Autodesk Inventor part; units mm, degrees
ref_plane "Work Plane2" through (0, 17.6708, -22.228) normal (0, 0, -1) x (0, 1, 0)
ref_plane "YZ Plane" through (0, 0, 0) normal (1, 0, 0) x (0, 1, 0)
ref_plane "XZ Plane" through (0, 0, 0) normal (0, 1, 0) x (-1, 0, 0)
ref_plane "Work Plane1" through (0, 0, 0) normal (0, 0, 1) x (1, 0, 0)
sketch "Sketch1" plane through (0, 0, 0) normal (0, 0, 1) x (1, 0, 0)
  arc A0 (18.9992, 41.108) -> (0, 60.0877) centre (-0.0008, 41.0877) ccw construction
  arc A1 (0, 22.1284) -> (18.9992, 41.108) centre (-0.0008, 41.1284) ccw construction
  arc A2 (44.3468, 60.0877) -> (25.3476, 41.108) centre (44.3476, 41.0877) ccw construction
  arc A3 (25.3476, 41.108) -> (44.3468, 22.1284) centre (44.3476, 41.1284) ccw construction
  line L0 (10.16, 73.6386) -> (5.7912, 73.6386) construction
  line L1 (0, 77.677) -> (0, 67.7202) construction
  line L2 (5.7912, 73.6386) -> (13.9012, 73.6386) construction
  line L3 (-25.35, 77.677) -> (-25.35, 84.027)
  line L4 (-25.35, -6.35) -> (-25.35, 0)
  line L5 (-25.35, 77.677) -> (-25.35, 0) construction
  arc A4 (-6.0324, 64.4924) -> (-6.0325, 17.7644) centre (-0.0008, 41.1284) ccw
  arc A5 (-6.0324, 64.4924) -> (-6.0325, 17.7644) centre (-0.0008, 41.1284) ccw
  arc A6 (-0.0008, 60.1276) -> (-0.0008, 22.1292) centre (-0.0008, 41.1284) ccw
  line L6 (-6.0324, 64.4924) -> (-6.0324, 73.6793)
  line L7 (10.16, 8.5775) -> (5.7912, 8.5775) construction
  line L8 (-6.0325, 8.5775) -> (-6.0325, 17.7644)
  line L9 (-0.0008, 73.6793) -> (-0.0008, 60.1276)
  line L10 (-0.0008, 8.5775) -> (-0.0008, 22.1292)
  line L11 (-6.0324, 73.6793) -> (-6.0324, 76.2193)
  line L12 (-6.0324, 76.2193) -> (0, 76.2193)
  line L13 (-0.0008, 73.6793) -> (0, 76.2193)
  line L14 (-6.0325, 8.5775) -> (-6.0325, 6.0375)
  line L15 (-6.0325, 6.0375) -> (-0.0008, 6.0375)
  line L16 (-0.0008, 6.0375) -> (-0.0008, 8.5775)
  point P0 (0, 0)
  dimension "d12" = 18.9992
  dimension "d13" = 24.13
  dimension "d19" = 6.0317
  dimension "d22" = 6.0317
  dimension "d23" = 0
  dimension "d24" = 0
  dimension "d44" = 2.54
  dimension "d45" = 2.54
ref_plane "Work Plane2" through (0, 17.6708, -22.228) normal (0, 0, -1) x (0, 1, 0)
extrude "Extrusion1" add sketch "Sketch1" against normal up to surface (22.228 mm away)
fillet "Fillet1" radius 3.175 1 edges at (-6.0324, 64.4924, -11.114)
fillet "Fillet2" radius 3.175 1 edges at (-6.0325, 17.7644, -11.114)
sketch "Sketch3" plane through (-6.0325, 8.5775, -22.228) normal (-1, 0, 0) x (0, 0, 1)
  circle A0 centre (5.08, 4.7016) radius 1.9304 construction
  circle A1 centre (17.148, 4.7016) radius 1.9304 construction
  circle A2 centre (17.148, 60.4409) radius 1.9304 construction
  circle A3 centre (5.08, 60.4409) radius 1.9304 construction
  line L0 (5.08, 4.0666) -> (5.08, 5.3366) construction
  line L1 (7.0104, 4.0666) -> (7.0104, 5.3366)
  line L2 (3.1496, 5.3366) -> (3.1496, 4.0666)
  arc A4 (3.1496, 4.0666) -> (7.0104, 4.0666) centre (5.08, 4.0666) ccw
  arc A5 (7.0104, 5.3366) -> (3.1496, 5.3366) centre (5.08, 5.3366) ccw
  point P0 (22.228, -8.5775)
  point P1 (5.08, 7.9375)
  dimension "d25" = 0.635
  dimension "d26" = 0.635
  dimension "d27" = 3.8608
extrude "Extrusion3" cut sketch "Sketch3" against normal through all both and the other way through all
sketch "Sketch4" plane through (-6.0325, 8.5775, -22.228) normal (-1, 0, 0) x (0, 0, 1)
  circle A0 centre (17.148, 4.7016) radius 1.9304 construction
  circle A1 centre (5.08, 60.4409) radius 1.9304 construction
  circle A2 centre (17.148, 60.4409) radius 1.9304 construction
  line L0 (17.148, 4.0666) -> (17.148, 5.3366) construction
  line L1 (19.0784, 4.0666) -> (19.0784, 5.3366)
  line L2 (15.2176, 5.3366) -> (15.2176, 4.0666)
  arc A3 (15.2176, 4.0666) -> (19.0784, 4.0666) centre (17.148, 4.0666) ccw
  arc A4 (19.0784, 5.3366) -> (15.2176, 5.3366) centre (17.148, 5.3366) ccw
  line L3 (5.08, 59.8059) -> (5.08, 61.0759) construction
  line L4 (7.0104, 59.8059) -> (7.0104, 61.0759)
  line L5 (3.1496, 61.0759) -> (3.1496, 59.8059)
  arc A5 (3.1496, 59.8059) -> (7.0104, 59.8059) centre (5.08, 59.8059) ccw
  arc A6 (7.0104, 61.0759) -> (3.1496, 61.0759) centre (5.08, 61.0759) ccw
  line L6 (17.148, 59.8059) -> (17.148, 61.0759) construction
  line L7 (19.0784, 59.8059) -> (19.0784, 61.0759)
  line L8 (15.2176, 61.0759) -> (15.2176, 59.8059)
  arc A7 (15.2176, 59.8059) -> (19.0784, 59.8059) centre (17.148, 59.8059) ccw
  arc A8 (19.0784, 61.0759) -> (15.2176, 61.0759) centre (17.148, 61.0759) ccw
  point P0 (22.228, -8.5775)
  point P1 (17.148, 4.7016)
  dimension "d30" = 0.635
  dimension "d31" = 0.635
  dimension "d32" = 0.635
  dimension "d33" = 0.635
  dimension "d34" = 0.635
  dimension "d35" = 0.635
  dimension "d36" = 3.8608
  dimension "d37" = 3.8608
  dimension "d38" = 3.8608
extrude "Extrusion4" cut sketch "Sketch4" against normal through all both and the other way through all
equation "\"d19\" = d18"
properties part number "motor mount cap"
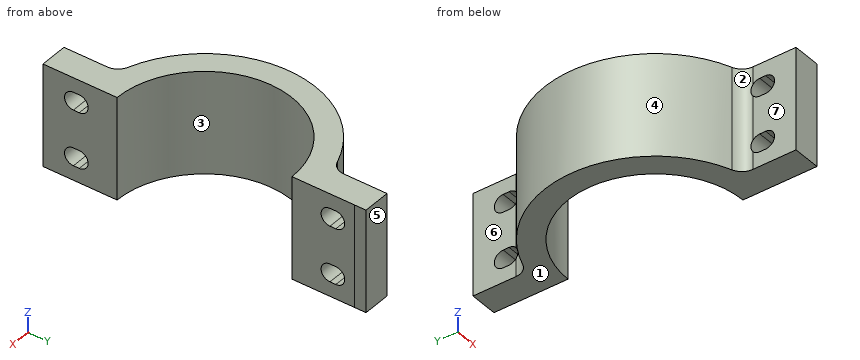
Read the model definition and answer for the solid it produces. Units are mm, in the model's axes. Face numbers are marked on the shaded views. A direction names the side the tool comes from. Round coordinates to 2 decimals unless told otherwise and drop trailing zeros. Order: outer loops, then holes, each group sorted by start corner. A loop starts at its lowest first (then second) coordinate and runs counter-clockwise, first axis right, second up. Notation, with made-up numbers: (60, -27.5) - (76, -27.5) arc R21 cw to (76, -9.5) - close; hole circle Ø10 at (-16.5, 17). An arc over 180 degrees is marked (long way). Use one line per item in the form item = value. Start each with the question number.
(1) Determine the mould class of the marked faces 1, 2, 3 and 4 for opening direction Y: +Y half, -Y half, draft (parallel to the pull), parting line (faces both ways), or undercut.
(2) For the marked faces 5, 6 and 7, determine the directions among +Z, -Z, +X, -X, +Y, -Y from which every point of the face is accessible in a straight line to the end or side of a thin tool.
(3) Flat-ended cylindrical pins translate along their axes: pin 1 Ø5 at (y, z) = (36, -2.5) entering from -X; pin 2 Ø7.5 at (y, z) = (72.5, -15) entering from -X; pin 3 Ø10 at (y, z) = (64, -20) entering from -X. Find the tip coordinate at first contact, or state that the pin passes through.
(4) The part is cut by section B-B (z = -5.08). Count the separate pieces of the cut face and the enclosed holes in it, then the cut area to 3 significant figures.
(5) Find the intervals of material crossed by line 1 along X through (y, z) = (9.5, -1.5); line 2 along Y through (x, z) = (-3.25, -14.5); line 3 along Y through (x, z) = (-13, -16.5), in increasing order. Write a range as from..to.
(6) The part is cut by section A-A (x = -3.5). Give the vertices of the cut face in (y, z).
(7) The part is cut by section D-D (y = 31.5). Give the vertices of the cut face in (x, z), then the cut area to 3 significant figures.
Checked values:
q1.face_1 = draft
q1.face_2 = -Y half
q1.face_3 = undercut
q1.face_4 = parting line
q2.face_5 = +Z, -Z, +X, -X, +Y
q2.face_6 = +Z, -Z, -X, +Y
q2.face_7 = +Z, -Z, -X, -Y
q3.pin_1 = -23.99
q3.pin_2 = -6.03
q3.pin_3 = -16.21
q4.separate_pieces = 3
q4.enclosed_holes = 0
q4.area = 423 mm^2
q5.line_1 = -6.03..0
q5.line_2 = 6.04..22.41, 59.85..76.22
q5.line_3 = 20.8..27.27, 54.98..61.46
q6.outline = (6.04, -22.23) - (22.45, -22.23) - (22.45, 0) - (6.04, 0) - close; (59.8, -22.23) - (76.22, -22.23) - (76.22, 0) - (59.8, 0) - close; hole (12.64, -19.08) - (13.91, -19.08) arc R1.93 ccw to (13.91, -15.22) - (12.64, -15.22) arc R1.93 ccw to start; hole (12.64, -7.01) - (13.91, -7.01) arc R1.93 ccw to (13.91, -3.15) - (12.64, -3.15) arc R1.93 ccw to start; hole (68.38, -19.08) - (69.65, -19.08) arc R1.93 ccw to (69.65, -15.22) - (68.38, -15.22) arc R1.93 ccw to start; hole (68.38, -7.01) - (69.65, -7.01) arc R1.93 ccw to (69.65, -3.15) - (68.38, -3.15) arc R1.93 ccw to start
q7.outline = (-22.13, -22.23) - (-16.38, -22.23) - (-16.38, 0) - (-22.13, 0) - close
q7.area = 128 mm^2
